Input: part model. Units: mm. Frame: model coordinates. Face numbers are marked on the shaded views. A direction names the side the tool comes from. Round coordinates to 2 decimals unless told otherwise and drop trailing zeros. Order: outer loops, then holes, each group sorted by start corner. A loop starts at its lowest first (then second) coordinate and runs counter-clockwise, first axis right, second up. Notation, with made-up numbers: M -7.5,26 L 8.5,26 A28 cw 8.5,60 Z; hole C -21,6 d8. An arc over 180 degrees is marked long. One line per question, with ' | ' between items.
```python
from build123d import *

# Parameters (mm, degrees)
SKETCH1_R           = 6
SKETCH1_R_2         = 4
BOSS_EXTRUDE1_DEPTH = 5
SKETCH2_R           = 6
SKETCH2_R_2         = 4
BOSS_EXTRUDE2_DEPTH = 5
BOSS_EXTRUDE3_DEPTH = 10


with BuildPart() as part:
    # Sketch1 → Boss-Extrude1 (new body)
    with BuildSketch(Plane(origin=(0, 0, 0), x_dir=(1, 0, 0), z_dir=(0, 1, 0))):
        with Locations(Location((1, 0, 0), (0, 0, 270))):
            Circle(SKETCH1_R)
        with Locations(Location((0, 0, 0), (0, 0, 270))):
            Circle(SKETCH1_R_2, mode=Mode.SUBTRACT)
    extrude(amount=BOSS_EXTRUDE1_DEPTH)

    # Sketch2 → Boss-Extrude2 (add)
    with BuildSketch(Plane(origin=(0, 5, 0), x_dir=(1, 0, 0), z_dir=(0, 1, 0))):
        with Locations(Location((-1, 0, 0), (0, 0, 80.405931773))):
            Circle(SKETCH2_R)
        with Locations(Location((0, 0, 0), (0, 0, 270))):
            Circle(SKETCH2_R_2, mode=Mode.SUBTRACT)
    extrude(amount=BOSS_EXTRUDE2_DEPTH)

    # Sketch3 → Boss-Extrude3 (add)
    with BuildSketch(Plane(origin=(0, 0, 0), x_dir=(1, 0, 0), z_dir=(0, 1, 0))):
        with BuildLine():
            Line((-2.5, 3.122498999), (-2.5, -3.122498999))
            ThreePointArc((-2.5, -3.122498999), (-4, 0), (-2.5, 3.122498999))
        make_face()
    extrude(amount=BOSS_EXTRUDE3_DEPTH)


solid = part.part
```
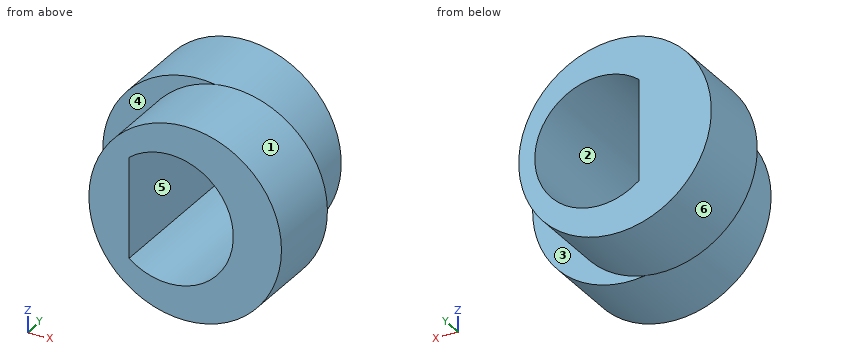
Item 1: First-contact query: pin 1 (1.9 mm diameter, centred on y = 7, z = 0, fed in from +X); pin 2 (6 mm diameter, centred on y = 6, z = -4, fed in from +X); pin 3 (1 mm diameter, centred on y = 1.5, z = 3.5, fed in from +X). Flat tips, straight axial feed; report the tip coordinate or a pass-through.
Report:
pin 1: x = 5 | pin 2: x = 6.88 | pin 3: x = 6.2
Item 2: Mould query, pull axis Z, two halves, no side actions, for the marked faces 1, 2 and 3. Classes: +Z half, -Z half, draft (parallel to the pull), parting line (faces both ways), or undercut.
Report:
face 1: parting line | face 2: undercut | face 3: draft
Item 3: Section query A-A, the plane z = 0. Return loops of the section in (x, y), plus the area to 3 significant figures.
Report:
outline: M -7,5 L -5,5 L -5,0 L -2.5,0 L -2.5,10 L -7,10 Z; M 4,0 L 7,0 L 7,5 L 5,5 L 5,10 L 4,10 Z | area: 55.0 mm²
Item 4: Access query for the marked faces 4, 5 and 6. Directions: +Z, -Z, +X, -X, +Y, -Y. A direction counts if a zero-diameter tool reaches every point of the face in a straight line with its end or side. Return the directions, or none.
Report:
face 4: -X, -Y | face 5: +Y, -Y | face 6: +Y
Item 5: Section query D-D, the plane x = -4.25. Return loops of the section in (y, z), plus the area to 3 significant figures.
Report:
outline: M 0,-2.9 L 5,-2.9 L 5,-5.04 L 10,-5.04 L 10,5.04 L 5,5.04 L 5,2.9 L 0,2.9 Z | area: 79.5 mm²
Item 6: Section query C-C, the plane y = 1.5. Return loops of the section in (x, z).
Report:
outline: C 1,0 d12; hole M -2.5,-3.12 A4 ccw long -2.5,3.12 Z
Item 7: Section query B-B, the plane x = 1. Return loops of the section in (y, z).
Report:
outline: M 0,-6 L 5,-6 L 5,-5.66 L 10,-5.66 L 10,-3.87 L 0,-3.87 Z; M 0,3.87 L 10,3.87 L 10,5.66 L 5,5.66 L 5,6 L 0,6 Z
Item 8: Line query: line 1 along Z through (x, y) = (-2, 2.5); line 2 along Y through (x, z) = (6.75, 0.5); line 3 along X through (y, z) = (7.5, 1.25). Output: solid intervals per line, ascending. Write a range as from..to.
Report:
line 1: -5.2..-3.46, 3.46..5.2 | line 2: 0..5 | line 3: -6.87..-2.5, 3.8..4.87
